Model file for the job. Use its own axes, mm. A direction names the side the tool comes from. Coordinates: 2 decimals unless noted, no trailing zeros. Loops run counter-clockwise (first coordinate to the right, second up) from the corner with the lowest first, then second, coordinate; pieces in that order, holes last. Notation, with made-up numbers: (-6, 35) -> (32, 35) arc R30 ccw to (32, 57) -> close; hole circle Ø9 at (4.25, -11). An arc over 180 degrees is marked (long way). Use one line per item in the form item = value.
```python
from build123d import *

# Parameters (mm, degrees)
BOSS_EXTRUDE1_START  = 36
SKETCH1_W            = 126
SKETCH1_H            = 98
BOSS_EXTRUDE1_DEPTH  = 2.4
BOSS_EXTRUDE2_START  = 37.9
SKETCH2_W            = 120.6
SKETCH2_H            = 92.6
BOSS_EXTRUDE2_DEPTH  = 4.5
BOSS_EXTRUDE3_START  = 38.4
SKETCH3_W            = 115.8
SKETCH3_H            = 87.8
BOSS_EXTRUDE3_DEPTH  = 5
BOSS_EXTRUDE4_START  = -60.3
SKETCH4_R            = 2.8
BOSS_EXTRUDE4_DEPTH  = 4.8
BOSS_EXTRUDE5_START  = -61
SKETCH5_R            = 1
BOSS_EXTRUDE5_DEPTH  = 6.5
BOSS_EXTRUDE6_START  = -60.3
SKETCH6_R            = 2.8
BOSS_EXTRUDE6_DEPTH  = 4.8
BOSS_EXTRUDE7_START  = -61
SKETCH7_R            = 1
BOSS_EXTRUDE7_DEPTH  = 6.5
BOSS_EXTRUDE8_START  = 55.5
SKETCH8_R            = 2.8
BOSS_EXTRUDE8_DEPTH  = 4.8
BOSS_EXTRUDE9_START  = 54.5
SKETCH9_R            = 1
BOSS_EXTRUDE9_DEPTH  = 6.5
BOSS_EXTRUDE10_START = 55.5
SKETCH10_R           = 2.8
BOSS_EXTRUDE10_DEPTH = 4.8
BOSS_EXTRUDE11_START = 54.5
SKETCH11_R           = 1
BOSS_EXTRUDE11_DEPTH = 6.5
BOSS_EXTRUDE12_START = 35
SKETCH12_R           = 1.5
BOSS_EXTRUDE12_DEPTH = 4.4
BOSS_EXTRUDE13_START = 35
SKETCH13_R           = 1.5
BOSS_EXTRUDE13_DEPTH = 4.4
BOSS_EXTRUDE14_START = 35
SKETCH14_R           = 1.5
BOSS_EXTRUDE14_DEPTH = 4.4
BOSS_EXTRUDE15_START = 35
SKETCH15_R           = 1.5
BOSS_EXTRUDE15_DEPTH = 4.4
BOSS_EXTRUDE16_START = 35
SKETCH16_R           = 1.5
BOSS_EXTRUDE16_DEPTH = 4.4
BOSS_EXTRUDE17_START = 35
SKETCH17_R           = 1.5
BOSS_EXTRUDE17_DEPTH = 4.4
BOSS_EXTRUDE18_START = 35
SKETCH18_R           = 1.5
BOSS_EXTRUDE18_DEPTH = 4.4
BOSS_EXTRUDE19_START = 35
SKETCH19_R           = 1.5
BOSS_EXTRUDE19_DEPTH = 4.4
BOSS_EXTRUDE20_START = 35
SKETCH20_R           = 1.5
BOSS_EXTRUDE20_DEPTH = 4.4
BOSS_EXTRUDE21_START = 38.4
SKETCH21_W           = 1.2
SKETCH21_H           = 33
BOSS_EXTRUDE21_DEPTH = 3
BOSS_EXTRUDE22_START = 38.4
SKETCH22_W           = 1.2
SKETCH22_H           = 33
BOSS_EXTRUDE22_DEPTH = 3
BOSS_EXTRUDE23_START = 38.4
SKETCH23_W           = 30.6
SKETCH23_H           = 1.2
BOSS_EXTRUDE23_DEPTH = 3
BOSS_EXTRUDE24_START = 38.4
SKETCH24_W           = 30.6
SKETCH24_H           = 1.2
BOSS_EXTRUDE24_DEPTH = 3
BOSS_EXTRUDE25_START = 35
SKETCH25_R           = 1.5
BOSS_EXTRUDE25_DEPTH = 4.4
BOSS_EXTRUDE26_START = 35
SKETCH26_R           = 1.5
BOSS_EXTRUDE26_DEPTH = 4.4


with BuildPart() as part:
    # Sketch1 → Boss-Extrude1 (new body)
    with BuildSketch(Plane.XY.offset(BOSS_EXTRUDE1_START)):
        with Locations((0, 109)):
            Rectangle(SKETCH1_W, SKETCH1_H)
    extrude(amount=BOSS_EXTRUDE1_DEPTH)

    # Sketch2 → Boss-Extrude2 (add)
    with BuildSketch(Plane.XY.offset(BOSS_EXTRUDE2_START)):
        with Locations((0, 109)):
            Rectangle(SKETCH2_W, SKETCH2_H)
    extrude(amount=BOSS_EXTRUDE2_DEPTH)


with BuildPart() as body_2:
    # Sketch3 → Boss-Extrude3 (new body)
    with BuildSketch(Plane.XY.offset(BOSS_EXTRUDE3_START)):
        with Locations((0, 109)):
            Rectangle(SKETCH3_W, SKETCH3_H)
    extrude(amount=BOSS_EXTRUDE3_DEPTH)


with BuildPart() as part_1:
    add(part.part)

    # Combine1: cut body 2
    add(body_2.part, mode=Mode.SUBTRACT)

    # Sketch4 → Boss-Extrude4 (add)
    with BuildSketch(Plane(origin=(0, 0, 0), x_dir=(0, 0, -1), z_dir=(1, 0, 0)).offset(BOSS_EXTRUDE4_START)):
        with Locations(Location((-41.5, 80, 0), (0, 0, 108.749340847))):
            Circle(SKETCH4_R)
    extrude(amount=BOSS_EXTRUDE4_DEPTH)


with BuildPart() as body_2_2:
    # Sketch5 → Boss-Extrude5 (new body)
    with BuildSketch(Plane(origin=(0, 0, 0), x_dir=(0, 0, -1), z_dir=(1, 0, 0)).offset(BOSS_EXTRUDE5_START)):
        with Locations((-41.5, 80)):
            Circle(SKETCH5_R)
    extrude(amount=BOSS_EXTRUDE5_DEPTH)


with BuildPart() as part_2:
    add(part_1.part)

    # Combine2: cut body 2 2
    add(body_2_2.part, mode=Mode.SUBTRACT)

    # Sketch6 → Boss-Extrude6 (add)
    with BuildSketch(Plane(origin=(0, 0, 0), x_dir=(0, 0, -1), z_dir=(1, 0, 0)).offset(BOSS_EXTRUDE6_START)):
        with Locations(Location((-41.5, 140, 0), (0, 0, 251.250659153))):
            Circle(SKETCH6_R)
    extrude(amount=BOSS_EXTRUDE6_DEPTH)


with BuildPart() as body_2_3:
    # Sketch7 → Boss-Extrude7 (new body)
    with BuildSketch(Plane(origin=(0, 0, 0), x_dir=(0, 0, -1), z_dir=(1, 0, 0)).offset(BOSS_EXTRUDE7_START)):
        with Locations((-41.5, 140)):
            Circle(SKETCH7_R)
    extrude(amount=BOSS_EXTRUDE7_DEPTH)


with BuildPart() as part_3:
    add(part_2.part)

    # Combine3: cut body 2 3
    add(body_2_3.part, mode=Mode.SUBTRACT)

    # Sketch8 → Boss-Extrude8 (add)
    with BuildSketch(Plane(origin=(0, 0, 0), x_dir=(0, 0, -1), z_dir=(1, 0, 0)).offset(BOSS_EXTRUDE8_START)):
        with Locations(Location((-41.5, 80, 0), (0, 0, 108.749340847))):
            Circle(SKETCH8_R)
    extrude(amount=BOSS_EXTRUDE8_DEPTH)


with BuildPart() as body_2_4:
    # Sketch9 → Boss-Extrude9 (new body)
    with BuildSketch(Plane(origin=(0, 0, 0), x_dir=(0, 0, -1), z_dir=(1, 0, 0)).offset(BOSS_EXTRUDE9_START)):
        with Locations((-41.5, 80)):
            Circle(SKETCH9_R)
    extrude(amount=BOSS_EXTRUDE9_DEPTH)


with BuildPart() as part_4:
    add(part_3.part)

    # Combine4: cut body 2 4
    add(body_2_4.part, mode=Mode.SUBTRACT)

    # Sketch10 → Boss-Extrude10 (add)
    with BuildSketch(Plane(origin=(0, 0, 0), x_dir=(0, 0, -1), z_dir=(1, 0, 0)).offset(BOSS_EXTRUDE10_START)):
        with Locations(Location((-41.5, 140, 0), (0, 0, 251.250659153))):
            Circle(SKETCH10_R)
    extrude(amount=BOSS_EXTRUDE10_DEPTH)


with BuildPart() as body_2_5:
    # Sketch11 → Boss-Extrude11 (new body)
    with BuildSketch(Plane(origin=(0, 0, 0), x_dir=(0, 0, -1), z_dir=(1, 0, 0)).offset(BOSS_EXTRUDE11_START)):
        with Locations((-41.5, 140)):
            Circle(SKETCH11_R)
    extrude(amount=BOSS_EXTRUDE11_DEPTH)


with BuildPart() as part_5:
    add(part_4.part)

    # Combine5: cut body 2 5
    add(body_2_5.part, mode=Mode.SUBTRACT)


with BuildPart() as body_2_6:
    # Sketch12 → Boss-Extrude12 (new body)
    with BuildSketch(Plane.XY.offset(BOSS_EXTRUDE12_START)):
        with Locations((-38, 88)):
            Circle(SKETCH12_R)
    extrude(amount=BOSS_EXTRUDE12_DEPTH)


with BuildPart() as part_6:
    add(part_5.part)

    # Combine6: cut body 2 6
    add(body_2_6.part, mode=Mode.SUBTRACT)


with BuildPart() as body_2_7:
    # Sketch13 → Boss-Extrude13 (new body)
    with BuildSketch(Plane.XY.offset(BOSS_EXTRUDE13_START)):
        with Locations((-38, 96)):
            Circle(SKETCH13_R)
    extrude(amount=BOSS_EXTRUDE13_DEPTH)


with BuildPart() as part_7:
    add(part_6.part)

    # Combine7: cut body 2 7
    add(body_2_7.part, mode=Mode.SUBTRACT)


with BuildPart() as body_2_8:
    # Sketch14 → Boss-Extrude14 (new body)
    with BuildSketch(Plane.XY.offset(BOSS_EXTRUDE14_START)):
        with Locations((-38, 104)):
            Circle(SKETCH14_R)
    extrude(amount=BOSS_EXTRUDE14_DEPTH)


with BuildPart() as part_8:
    add(part_7.part)

    # Combine8: cut body 2 8
    add(body_2_8.part, mode=Mode.SUBTRACT)


with BuildPart() as body_2_9:
    # Sketch15 → Boss-Extrude15 (new body)
    with BuildSketch(Plane.XY.offset(BOSS_EXTRUDE15_START)):
        with Locations((-30, 88)):
            Circle(SKETCH15_R)
    extrude(amount=BOSS_EXTRUDE15_DEPTH)


with BuildPart() as part_9:
    add(part_8.part)

    # Combine9: cut body 2 9
    add(body_2_9.part, mode=Mode.SUBTRACT)


with BuildPart() as body_2_10:
    # Sketch16 → Boss-Extrude16 (new body)
    with BuildSketch(Plane.XY.offset(BOSS_EXTRUDE16_START)):
        with Locations((-30, 96)):
            Circle(SKETCH16_R)
    extrude(amount=BOSS_EXTRUDE16_DEPTH)


with BuildPart() as part_10:
    add(part_9.part)

    # Combine10: cut body 2 10
    add(body_2_10.part, mode=Mode.SUBTRACT)


with BuildPart() as body_2_11:
    # Sketch17 → Boss-Extrude17 (new body)
    with BuildSketch(Plane.XY.offset(BOSS_EXTRUDE17_START)):
        with Locations((-30, 104)):
            Circle(SKETCH17_R)
    extrude(amount=BOSS_EXTRUDE17_DEPTH)


with BuildPart() as part_11:
    add(part_10.part)

    # Combine11: cut body 2 11
    add(body_2_11.part, mode=Mode.SUBTRACT)


with BuildPart() as body_2_12:
    # Sketch18 → Boss-Extrude18 (new body)
    with BuildSketch(Plane.XY.offset(BOSS_EXTRUDE18_START)):
        with Locations((-22, 88)):
            Circle(SKETCH18_R)
    extrude(amount=BOSS_EXTRUDE18_DEPTH)


with BuildPart() as part_12:
    add(part_11.part)

    # Combine12: cut body 2 12
    add(body_2_12.part, mode=Mode.SUBTRACT)


with BuildPart() as body_2_13:
    # Sketch19 → Boss-Extrude19 (new body)
    with BuildSketch(Plane.XY.offset(BOSS_EXTRUDE19_START)):
        with Locations((-22, 96)):
            Circle(SKETCH19_R)
    extrude(amount=BOSS_EXTRUDE19_DEPTH)


with BuildPart() as part_13:
    add(part_12.part)

    # Combine13: cut body 2 13
    add(body_2_13.part, mode=Mode.SUBTRACT)


with BuildPart() as body_2_14:
    # Sketch20 → Boss-Extrude20 (new body)
    with BuildSketch(Plane.XY.offset(BOSS_EXTRUDE20_START)):
        with Locations((-22, 104)):
            Circle(SKETCH20_R)
    extrude(amount=BOSS_EXTRUDE20_DEPTH)


with BuildPart() as part_14:
    add(part_13.part)

    # Combine14: cut body 2 14
    add(body_2_14.part, mode=Mode.SUBTRACT)

    # Sketch21 → Boss-Extrude21 (add)
    with BuildSketch(Plane.XY.offset(BOSS_EXTRUDE21_START)):
        with Locations((-45.9, 95.5)):
            Rectangle(SKETCH21_W, SKETCH21_H)
    extrude(amount=BOSS_EXTRUDE21_DEPTH)

    # Sketch22 → Boss-Extrude22 (add)
    with BuildSketch(Plane.XY.offset(BOSS_EXTRUDE22_START)):
        with Locations((-14.1, 95.5)):
            Rectangle(SKETCH22_W, SKETCH22_H)
    extrude(amount=BOSS_EXTRUDE22_DEPTH)

    # Sketch23 → Boss-Extrude23 (add)
    with BuildSketch(Plane.XY.offset(BOSS_EXTRUDE23_START)):
        with Locations((-30, 112.9)):
            Rectangle(SKETCH23_W, SKETCH23_H)
    extrude(amount=BOSS_EXTRUDE23_DEPTH)

    # Sketch24 → Boss-Extrude24 (add)
    with BuildSketch(Plane.XY.offset(BOSS_EXTRUDE24_START)):
        with Locations((-30, 78.1)):
            Rectangle(SKETCH24_W, SKETCH24_H)
    extrude(amount=BOSS_EXTRUDE24_DEPTH)


with BuildPart() as body_2_15:
    # Sketch25 → Boss-Extrude25 (new body)
    with BuildSketch(Plane.XY.offset(BOSS_EXTRUDE25_START)):
        with Locations((51.5, 98.5)):
            Circle(SKETCH25_R)
    extrude(amount=BOSS_EXTRUDE25_DEPTH)


with BuildPart() as part_15:
    add(part_14.part)

    # Combine15: cut body 2 15
    add(body_2_15.part, mode=Mode.SUBTRACT)


with BuildPart() as body_2_16:
    # Sketch26 → Boss-Extrude26 (new body)
    with BuildSketch(Plane.XY.offset(BOSS_EXTRUDE26_START)):
        with Locations((51.5, 90.8)):
            Circle(SKETCH26_R)
    extrude(amount=BOSS_EXTRUDE26_DEPTH)


with BuildPart() as part_16:
    add(part_15.part)

    # Combine16: cut body 2 16
    add(body_2_16.part, mode=Mode.SUBTRACT)


solid = part_16.part
```
Q1. Band-saw the part on C-C, the plane y = 134. Write the cut outline in (x, z), and give its area (3 significant figures).
Result:
outline = (-63, 36) -> (63, 36) -> (63, 38.4) -> (60.3, 38.4) -> (60.3, 42.4) -> (57.9, 42.4) -> (57.9, 38.4) -> (-57.9, 38.4) -> (-57.9, 42.4) -> (-60.3, 42.4) -> (-60.3, 38.4) -> (-63, 38.4) -> close
area = 322 mm2
Q2. Mould opens along Y. For faces 1 (the face through (55.5, 80, 40)), 2 (the face through (-9.2, 153.2, 42.4)), 3 (the face through (-1, 60, 37)) say: released by +Y, released by -Y, zero draft, split by the parting line, or undercut.
Result:
face_1 = undercut
face_2 = zero draft
face_3 = released by -Y
Q3. Wall check: line 1 along X through (y, z) = (108.5, 40); line 2 along Y through (x, z) = (-22, 36.5); line 3 along Y through (x, z) = (-57.45, 41.5). Give the ranges that are in metal, low to high.
Result:
line_1 = -60.3 to -57.9, -46.5 to -45.3, -14.7 to -13.5, 57.9 to 60.3
line_2 = 60 to 86.5, 89.5 to 94.5, 97.5 to 102.5, 105.5 to 158
line_3 = 62.7 to 65.1, 77.2 to 79, 81 to 82.8, 137.2 to 139, 141 to 142.8, 152.9 to 155.3
Q4. Pin check, flat tips, straight feed: pin 1 Ø1.6 at (y, z) = (80, 41.5) entering from -X; pin 2 Ø0.7 at (x, y) = (59, 101.5) entering from +Z; pin 3 Ø1 at (x, z) = (-14.5, 40.5) entering from -Y. Stop position of each tip, or through.
Result:
pin_1 = -46.5
pin_2 = 42.4
pin_3 = 62.7
Q5. Band-saw the part on A-A, the plane x = -30. State how many separate pieces and enclosed holes the cut face has, and give its area (3 significant figures).
Result:
separate_pieces = 4
enclosed_holes = 0
area = 240 mm2
Q6. Band-saw the part on D-D, the plane x = 0. Write the cut outline in (y, z), and give its area (3 significant figures).
Result:
outline = (60, 36) -> (158, 36) -> (158, 38.4) -> (155.3, 38.4) -> (155.3, 42.4) -> (152.9, 42.4) -> (152.9, 38.4) -> (65.1, 38.4) -> (65.1, 42.4) -> (62.7, 42.4) -> (62.7, 38.4) -> (60, 38.4) -> close
area = 254 mm2
Q7. Which spindle directions (+Z, -Z, +X, -X, +Y, -Y) get a long thin tool onto all of the face, cutting with end or side? Do faces 4 (the face through (60.3, 109, 40)), 5 (the face through (-30, 112.3, 40)), 6 (the face through (-57.4, 78.76, 44.01)), 7 (the face through (59, 110, 42.4)), 8 (the face through (-9.2, 64.6, 42.4)). Say none if no direction does.
Result:
face_4 = +Z, +X, +Y, -Y
face_5 = +Z
face_6 = none
face_7 = +Z, +X, -X
face_8 = +Z, +X, -X, -Y
